from build123d import *

# Parameters (mm, degrees)
F0_W     = 95.8645157516
F0_H     = 76.322901994
F1_DEPTH = 51.562
F2_W     = 74.2949992418
F2_H     = 35.2117735893
F3_DEPTH = 73.152
F4_R     = 7.4407227367
F5_DEPTH = 53.34
F6_W     = 42.9546777159
F6_H     = 31.5246768296
F7_DEPTH = 57.912


with BuildPart() as f1:
    # F0 (on Front) → F1 (new body)
    with BuildSketch(Plane.XZ):
        with Locations((-1.3826619834, 3.4105647355)):
            Rectangle(F0_W, F0_H)
    extrude(amount=-F1_DEPTH)

    # F2 (on Top) → F3 (cut)
    with BuildSketch(Plane.XY):
        with Locations((-2.9496774077, 27.4688703939)):
            Rectangle(F2_W, F2_H)
    extrude(amount=F3_DEPTH, mode=Mode.SUBTRACT)

    # F4 (on Right) → F5 (cut, symmetric)
    with BuildSketch(Plane.YZ):
        with Locations((27.929758653, 9.309919551)):
            Circle(F4_R)
    extrude(amount=F5_DEPTH, both=True, mode=Mode.SUBTRACT)

    # F6 (on face) → F7 (cut)
    with BuildSketch(Plane.XZ):
        with Locations((3.871451132, 25.8096773177)):
            Rectangle(F6_W, F6_H)
    extrude(amount=-F7_DEPTH, mode=Mode.SUBTRACT)


solid = f1.part
CAD build for the part. Positions are in the model's coordinates, mm. A direction names the side the tool comes from. Coordinates: 2 decimals unless noted, no trailing zeros. Write each loop counter-clockwise with the first axis right and the second up, starting at its lowest first coordinate (ties: lowest second). Pieces come first, ordered by that corner, then holes. Notation, with made-up numbers: M 87,54 L 137,54 A34 cw 137,92 Z; hole C 2,66 d11. An arc over 180 degrees is marked long. Return JSON: item names as keys, results as strings.
Item 1: Which spindle directions (+Z, -Z, +X, -X, +Y, -Y) get a long thin tool onto all of the face, cutting with end or side? Do faces 4 (the flat face through (-41, 25, 41.572)), 5 (the flat face through (25.349, 48, 26)), 6 (the flat face through (34.198, 27, 20)). Say none if no direction does.
Findings below:
{"face 4": "+Z, +X, -X, +Y, -Y", "face 5": "+Z, +Y, -Y", "face 6": "+Z"}
Item 2: Probe line 1 (X direction, y = 8, z = 37.5); line 2 (X direction, y = 35, z = 31); line 3 (Y direction, x = -28, z = 3). List the from-to ranges inside material, lowest first. Write a range as from..to.
Findings below:
{"line 1": "x = -49.31..-17.61, 25.35..46.55", "line 2": "x = -49.31..-40.1, 34.2..46.55", "line 3": "y = 0..9.86, 45.07..51.56"}
Item 3: Slice it at D-D, the plane x = 36.5. Write the cut outline in (y, z).
Findings below:
{"outline": "M 0,-34.75 L 51.56,-34.75 L 51.56,41.57 L 0,41.57 Z; hole C 27.93,9.31 d14.88"}
Item 4: Slice it at A-A, the plane z = 23.5. Write the cut outline in (x, y), and give its area (3 significant figures).
Findings below:
{"outline": "M -49.31,0 L -17.61,0 L -17.61,9.86 L -40.1,9.86 L -40.1,45.07 L -17.61,45.07 L -17.61,51.56 L -49.31,51.56 Z; M 25.35,0 L 46.55,0 L 46.55,51.56 L 25.35,51.56 L 25.35,45.07 L 34.2,45.07 L 34.2,9.86 L 25.35,9.86 Z", "area": "1,620 mm2"}
Item 5: Drop a flat-ended pin along its axis: pin 1 Ø11 at (x, y) = (-4.5, 4.5) entering from +Z. Give the stop position or say it passes through.
Findings below:
{"pin 1": "stops at z = 10.05"}
Item 6: Two-plate mould, pull along Y, no slides. Class faces 1 (the flat face through (-2, 51.562, -5)), 2 (the flat face through (-40.097, 27, 20)), 3 (the flat face through (-17.606, 48, 26)): +Y half, -Y half, draft (parallel to the pull), parting line (faces both ways), or undercut.
Findings below:
{"face 1": "+Y half", "face 2": "undercut", "face 3": "draft"}
Item 7: Slice it at B-B, the plane y = 33. Write the cut outline in (x, z).
Findings below:
{"outline": "M -49.31,-34.75 L 46.55,-34.75 L 46.55,3.86 L 34.2,3.86 L 34.2,0 L -40.1,0 L -40.1,3.86 L -49.31,3.86 Z; M -49.31,14.76 L -40.1,14.76 L -40.1,41.57 L -49.31,41.57 Z; M 34.2,14.76 L 46.55,14.76 L 46.55,41.57 L 34.2,41.57 Z"}
Item 8: Slice it at C-C, the plane y = 39. Write the cut outline in (x, z).
Findings below:
{"outline": "M -49.31,-34.75 L 46.55,-34.75 L 46.55,41.57 L 34.2,41.57 L 34.2,0 L -40.1,0 L -40.1,41.57 L -49.31,41.57 Z"}
